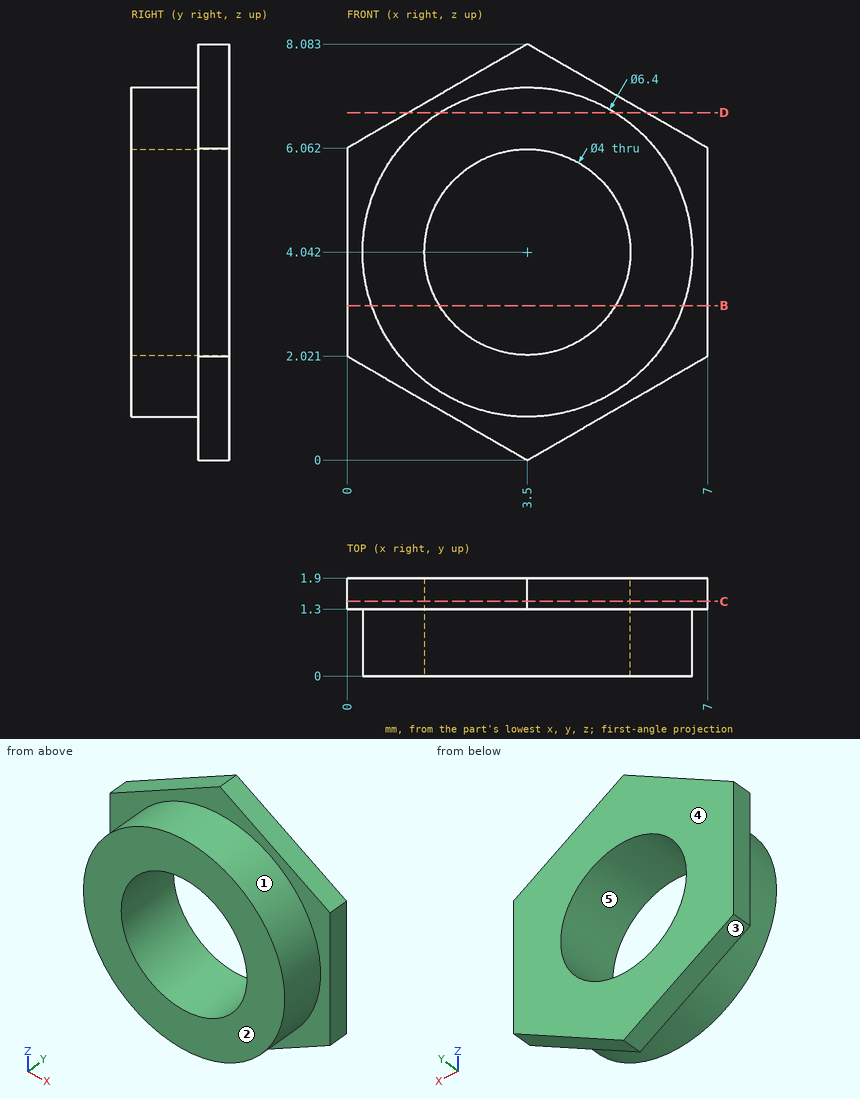
Part print with two shaded views. Sizes in mm from the minimum x, y, z corner. A direction names the side the tool comes from. Give positions to 0.01 mm unless a question says otherwise; leave off trailing zeros. Order: outer loops, then holes, each group sorted by start corner. A loop starts at its lowest first (then second) coordinate and runs counter-clockwise, first axis right, second up.
1) Saw through at C-C, the plane y = 1.45. Write the cut outline in (x, z).
2) Saw through at B-B, the plane z = 3. Write the cut outline in (x, y) (1 decimal).
3) Mould opens along Z. For the marked faces 3, 4 and 5 say: +Z half, -Z half, draft (parallel to the pull), parting line (faces both ways), or undercut.
4) Wall check: probe 1 along Z at (x, y) = (3.5, 0.9); probe 2 along X at (y, z) = (1.85, 4); probe 3 along X at (y, z) = (1, 4.25). Give the ranges that are in metal, low to high.
5) 3-axis set-ups, long thin cutter, end or side, ignore diameter. For the marked faces 1 and 2: which of +Z, -Z, +X, -X, +Y, -Y reach the whole face in a straight line?
6) Pin check, flat tip, straight feed: pin 1 (4 mm diameter, centred on x = 3.5, z = 3, fed in from +Y). Stop position of the tip, or through.
7) Saw through at D-D, the plane z = 6.75. Write the cut outline in (x, y) (1 decimal).
Computed:
1. outline: (0, 2.02) - (3.5, 0) - (7, 2.02) - (7, 6.06) - (3.5, 8.08) - (0, 6.06) - close; hole circle Ø4 at (3.5, 4.04)
2. outline: (0, 1.3) - (0.5, 1.3) - (0.5, 0) - (1.8, 0) - (1.8, 1.9) - (0, 1.9) - close; (5.2, 0) - (6.5, 0) - (6.5, 1.3) - (7, 1.3) - (7, 1.9) - (5.2, 1.9) - close
3. face 3: -Z half
3. face 4: draft
3. face 5: undercut
4. probe 1: z = 0.84 to 2.04, 6.04 to 7.24
4. probe 2: x = 0 to 1.5, 5.5 to 7
4. probe 3: x = 0.31 to 1.51, 5.49 to 6.69
5. face 1: -Y
5. face 2: +Z, -Z, +X, -X, -Y
6. pin 1: stops at y = 1.9
7. outline: (1.2, 1.3) - (1.8, 1.3) - (1.8, 0) - (5.2, 0) - (5.2, 1.3) - (5.8, 1.3) - (5.8, 1.9) - (1.2, 1.9) - close
